Geometry: final body of the model. Coordinates: model frame, mm. A direction names the side the tool comes from. Give positions to 0.01 mm unless a question says otherwise; leave off trailing zeros. Loops run counter-clockwise (first coordinate to the right, second up) from the corner with the lowest first, then second, coordinate; pieces in that order, holes last.
1. Section C-C, the plane x = -25. Output: boundary loops of the cut face in (y, z), then the cut area to 3 significant figures.
2. Access query for faces 5 (the face through (36, 11, -10)), 6 (the face through (-34, 9, 0)). Directions: +Z, -Z, +X, -X, +Y, -Y. A direction counts if a zero-diameter tool reaches every point of the face in a straight line with its end or side. Return the directions, or none.
3. Section D-D, the plane z = -25. Output: boundary loops of the cut face in (x, y), then the cut area to 3 significant figures.
4. Section A-A, the plane z = -10. Output: boundary loops of the cut face in (x, y), then the cut area to 3 significant figures.
5. Draft query along Y for faces 1 (the face through (9, 0, 14)), 2 (the face through (-35.972, 10.352, 21.474)), 3 (the face through (-36, 14, 0)), 4 (the face through (-38, 7, 0)). Return one class per face: +Y half, -Y half, draft (parallel to the pull), parting line (faces both ways), or undercut.
6. Material intervals for line 1 along X through (y, z) = (12.5, -14); line 2 along Y through (x, z) = (11.5, -27); line 3 along Y through (x, z) = (-35, 20), sorted ascending.
7. First-contact query: P1, Ø4.5, axis at x = 0, z = -25, coming from the +Y side. Flat tip, straight axial feed; report the tip coordinate or a pass-through.
8. Section B-B, the plane x = 0. Output: boundary loops of the cut face in (y, z).
from build123d import *

# Parameters (mm, degrees)
EXTRUDE_1_DEPTH     = 30
CUT_EXTRUDE_1_REACH = 84.898
SKETCH_2_R          = 2
SKETCH_3_R          = 16
SKETCH_3_R_2        = 2
CUT_EXTRUDE_2_DEPTH = 4


with BuildPart() as part:
    # 草图1 → 凸台-拉伸1 (new, symmetric)
    with BuildSketch(Plane.XY):
        Polygon((38, 0), (-38, 0), (-38, 14), (-34, 14), (-34, 4), (34, 4), (34, 14), (38, 14), align=None)
    extrude(amount=EXTRUDE_1_DEPTH, both=True)

    # 切除-拉伸1: up to this face of the body (flat: up to its plane)
    cut_extrude_1_end = Plane(part.part.faces().sort_by_distance((-38, 7, 0))[0])
    # 草图2 → 切除-拉伸1 (cut, up to the picked face)
    with BuildSketch(Plane(origin=(38, 0, 0), x_dir=(0, 0, -1), z_dir=(1, 0, 0)), mode=Mode.PRIVATE) as cut_extrude_1_sk1:
        with Locations((-20, 9)):
            Circle(SKETCH_2_R)
    cut_extrude_1_tool1 = split(extrude(cut_extrude_1_sk1.sketch, amount=-CUT_EXTRUDE_1_REACH, mode=Mode.PRIVATE), bisect_by=cut_extrude_1_end, keep=Keep.BOTH, mode=Mode.PRIVATE)
    # 草图2 → 切除-拉伸1 (cut, up to the picked face)
    with BuildSketch(Plane(origin=(38, 0, 0), x_dir=(0, 0, -1), z_dir=(1, 0, 0)), mode=Mode.PRIVATE) as cut_extrude_1_sk2:
        with Locations((-10, 9)):
            Circle(SKETCH_2_R)
    cut_extrude_1_tool2 = split(extrude(cut_extrude_1_sk2.sketch, amount=-CUT_EXTRUDE_1_REACH, mode=Mode.PRIVATE), bisect_by=cut_extrude_1_end, keep=Keep.BOTH, mode=Mode.PRIVATE)
    # 草图2 → 切除-拉伸1 (cut, up to the picked face)
    with BuildSketch(Plane(origin=(38, 0, 0), x_dir=(0, 0, -1), z_dir=(1, 0, 0)), mode=Mode.PRIVATE) as cut_extrude_1_sk3:
        with Locations((10, 9)):
            Circle(SKETCH_2_R)
    cut_extrude_1_tool3 = split(extrude(cut_extrude_1_sk3.sketch, amount=-CUT_EXTRUDE_1_REACH, mode=Mode.PRIVATE), bisect_by=cut_extrude_1_end, keep=Keep.BOTH, mode=Mode.PRIVATE)
    # 草图2 → 切除-拉伸1 (cut, up to the picked face)
    with BuildSketch(Plane(origin=(38, 0, 0), x_dir=(0, 0, -1), z_dir=(1, 0, 0)), mode=Mode.PRIVATE) as cut_extrude_1_sk4:
        with Locations((20, 9)):
            Circle(SKETCH_2_R)
    cut_extrude_1_tool4 = split(extrude(cut_extrude_1_sk4.sketch, amount=-CUT_EXTRUDE_1_REACH, mode=Mode.PRIVATE), bisect_by=cut_extrude_1_end, keep=Keep.BOTH, mode=Mode.PRIVATE)
    add(cut_extrude_1_tool1.solids().sort_by(Axis((38, 9, 20), (-1, 0, 0)))[0], mode=Mode.SUBTRACT)
    add(cut_extrude_1_tool2.solids().sort_by(Axis((38, 9, 10), (-1, 0, 0)))[0], mode=Mode.SUBTRACT)
    add(cut_extrude_1_tool3.solids().sort_by(Axis((38, 9, -10), (-1, 0, 0)))[0], mode=Mode.SUBTRACT)
    add(cut_extrude_1_tool4.solids().sort_by(Axis((38, 9, -20), (-1, 0, 0)))[0], mode=Mode.SUBTRACT)

    # 草图3 → 切除-拉伸2 (cut)
    with BuildSketch(Plane(origin=(0, 4, 0), x_dir=(1, 0, 0), z_dir=(0, 1, 0))):
        with Locations(Location((0, 0, 0), (0, 0, 270))):
            Circle(SKETCH_3_R)
        with Locations(Location((0, 25, 0), (0, 0, 270))):
            Circle(SKETCH_3_R_2)
        with Locations(Location((25, 0, 0), (0, 0, 270))):
            Circle(SKETCH_3_R_2)
        with Locations(Location((0, -25, 0), (0, 0, 270))):
            Circle(SKETCH_3_R_2)
        with Locations(Location((-25, 0, 0), (0, 0, 270))):
            Circle(SKETCH_3_R_2)
    extrude(amount=-CUT_EXTRUDE_2_DEPTH, mode=Mode.SUBTRACT)


solid = part.part
Answers below:
1. outline: (0, -30) - (4, -30) - (4, -2) - (0, -2) - close; (0, 2) - (4, 2) - (4, 30) - (0, 30) - close
1. area: 224 mm2
2. face 5: +X, -X
2. face 6: +Z, -Z, +Y
3. outline: (-38, 0) - (-2, 0) - (-2, 4) - (-34, 4) - (-34, 14) - (-38, 14) - close; (2, 0) - (38, 0) - (38, 14) - (34, 14) - (34, 4) - (2, 4) - close
3. area: 368 mm2
4. outline: (-38, 0) - (-12.49, 0) - (-12.49, 4) - (-34, 4) - (-34, 7) - (-38, 7) - close; (-38, 11) - (-34, 11) - (-34, 14) - (-38, 14) - close; (12.49, 0) - (38, 0) - (38, 7) - (34, 7) - (34, 4) - (12.49, 4) - close; (34, 11) - (38, 11) - (38, 14) - (34, 14) - close
4. area: 252 mm2
5. face 1: -Y half
5. face 2: undercut
5. face 3: +Y half
5. face 4: draft
6. line 1: x = -38 to -34, 34 to 38
6. line 2: y = 0 to 4
6. line 3: y = 0 to 7, 11 to 14
7. P1: stops at y = 4
8. outline: (0, -30) - (4, -30) - (4, -27) - (0, -27) - close; (0, -23) - (4, -23) - (4, -16) - (0, -16) - close; (0, 16) - (4, 16) - (4, 23) - (0, 23) - close; (0, 27) - (4, 27) - (4, 30) - (0, 30) - close
